Build history of the part. All positions in model axes, mm. A direction names the side the tool comes from. Round coordinates to 2 decimals unless told otherwise and drop trailing zeros. Loops run counter-clockwise (first coordinate to the right, second up) from the corner with the lowest first, then second, coordinate; pieces in that order, holes last.
Autodesk Inventor part; units mm, degrees
ref_plane "Arbeitsebene1" through (5, -3, 0) normal (0, 1, 0) x (-1, 0, 0)
ref_plane "YZ Plane" through (0, 0, 0) normal (1, 0, 0) x (0, 1, 0)
ref_plane "XY Plane" through (0, 0, 0) normal (0, 0, 1) x (1, 0, 0)
sketch "Skizze1" plane through (0, 0, 0) normal (0, 0, 1) x (1, 0, 0)
  line L0 (0, -0.6) -> (0, 3.6)
  line L1 (-2, 0) -> (12, 0)
  line L2 (0, 0) -> (10, 0)
  line L3 (10, 0) -> (10, 3)
  line L4 (10, 3) -> (0, 3)
  line L5 (0, 3) -> (0, 0)
  dimension "d1" = 10
  dimension "d2" = 6
revolve "Umdrehung1" add sketch "Skizze1" angle 360 about axis through (-10, 0, 0) along (1, 0, 0)
ref_plane "Arbeitsebene1" through (5, -3, 0) normal (0, 1, 0) x (-1, 0, 0)
sketch "Skizze2" plane through (5, -3, 0) normal (0, 1, 0) x (-1, 0, 0)
  line L0 (5, 3) -> (5, -3)
  line L1 (-5, 3) -> (-5, -3)
  line L2 (5, -3) -> (-5, -3)
  line L3 (5, 3) -> (-5, 3)
  line L4 (1.5, 3) -> (1.5, 1.5)
  line L5 (1.5, 1.5) -> (-5, 1.5)
  line L6 (-5, -1.5) -> (1.5, -1.5)
  line L7 (1.5, -1.5) -> (1.5, -3)
  line L8 (-5, 1.5) -> (-5, 3)
  line L9 (-5, 3) -> (1.5, 3)
  line L10 (-5, 3) -> (-5, -3)
  line L11 (-5, -1.5) -> (-5, -3)
  line L12 (-5, -3) -> (1.5, -3)
  dimension "d4" = 1.5
  dimension "d5" = 1.5
  dimension "d6" = 3.5
extrude "Extrusion1" cut sketch "Skizze2" along normal through all contours L4 L5 L1 L3 | L2 L1 L6 L7
chamfer "Fase1" distance 1.5 angle 33 1 edges at (0, -3, 0) measured on face at (4.5, -2.8079, -1.0563)
sketch "Skizze3" plane through (3.5, 2.5981, 1.5) normal (0, 0, 1) x (1, 0, 0)
  line L0 (6.5, 0) -> (6.5, -5.1962) construction
  arc A0 (3.5, -5.5981) -> (3.5, 0.4019) centre (3.5, -2.5981) ccw
  line L1 (6.5, 0) -> (6.5, 0.4019)
  line L2 (3.5, 0.4019) -> (7.092, 0.4019)
  line L3 (-2, 0.4019) -> (6.5, 0.4019)
  line L4 (7.092, 0.4019) -> (7.092, -5.5981)
  line L5 (7.092, -5.5981) -> (3.5, -5.5981)
  line L6 (-5.6184, -5.5981) -> (9.2105, -5.5981)
  point P0 (-3.5, -2.5981)
  point P1 (6.5, -5.5981)
  dimension "d13" = 3
  dimension "d14" = 3.592
extrude "Extrusion2" cut sketch "Skizze3" against normal through all
sketch "Skizze4" plane through (3.5, -2.5981, 1.5) normal (0, 0, 1) x (1, 0, 0)
  arc A0 (5, 0) -> (5, 5.1962) centre (3.5, 2.5981) ccw
  point P0 (-3.5, 2.5981)
hole "Bohrung1" at (7, 0, 1.5) at (7, 0, 1.5) direction (0, 0, -1) diameter 3 depth 3 tip angle 118
sketch "Skizze7" plane through (0, 0, 0) normal (-1, 0, 0) x (0, 0, 1)
  arc A0 (1.5, 2.5981) -> (-1.5, 2.5981) centre (0, 0) ccw
  circle A1 centre (0, 0) radius 3 construction
  line L0 (-1.5, 2.5981) -> (-1.5, 4)
  line L1 (-1.5, 4) -> (1.5, 4)
  line L2 (1.5, 4) -> (1.5, 2.5981)
  line L3 (0, -4.5424) -> (0, 5.5632)
  dimension "d25" = 1.5
  dimension "d26" = 3
  dimension "d27" = 4
sketch "Skizze8" plane through (3.5, -2.5981, 1.5) normal (0, 0, 1) x (1, 0, 0)
  line L0 (-2, 5.5981) -> (3.5, 5.5981)
  line L1 (3.5, 5.5981) -> (-3.5, 5.5981)
  arc A0 (5, 0) -> (5, 5.1962) centre (3.5, 2.5981) ccw
  arc A1 (3.5, -0.4019) -> (3.5, 5.5981) centre (3.5, 2.5981) ccw
  line L2 (-2, -0.4019) -> (3.5, -0.4019)
  line L3 (3.5, -0.4019) -> (-2.8962, -0.4019)
  point P0 (-3.5, 2.5981)
sweep "Sweeping2" cut profiles "Skizze7" path "Skizze8" path curves L1 A1 L3
sketch "Skizze9" plane through (0, 0, 0) normal (-1, 0, 0) x (0, 0, 1)
  point P0 (0, 0)
  point P1 (0, 0)
hole "Bohrung2" at (0, 0, 0) direction (1, 0, 0) diameter 2.459 depth 4 tip angle 118
properties part number "Stangenkopf"
(1) Slice it at C-C on x = 5. List the corners of the cut face in (y, z).
Responses:
outline: (-2.6, -1.5) - (2.6, -1.5) arc R3 ccw to (2.6, 1.5) - (-2.6, 1.5) arc R3 ccw to start
(2) Pull direction Y, two halves, no side cores. Call faces 4 (the face through (3.6, 2.86, -0.9)), 5 (the face through (2.028, 0.748, -0.976)), 6 (the face through (0, 1, -1)): +Y half, -Y half, draft (parallel to the pull), parting line (faces both ways), or undercut.
Responses:
face 4: parting line
face 5: undercut
face 6: draft
(3) Pin check, flat tips, straight feed: P1, Ø1.2, axis at y = 0.5, z = 2, coming from the +X side; P2, Ø2.5, axis at x = 6, y = -1, coming from the -Z side; P3, Ø3, axis at x = 8.5, z = -1, coming from the +Y side. Stop position of each tip, or through.
Responses:
P1: stops at x = 9.62
P2: stops at z = -1.5
P3: stops at y = 2.98
(4) Slice it at B-B on x = 2.5. List the corners of the cut face in (y, z).
Responses:
outline: circle Ø6 at (0, 0); hole circle Ø2.46 at (0, 0)
(5) Which spindle directions (+Z, -Z, +X, -X, +Y, -Y) get a long thin tool onto all of the face, cutting with end or side? Do faces 1 (the face through (4.61, 0.064, 0.204)), 2 (the face through (5, 0, 1.5)), 3 (the face through (5, 0, -1.5)). Say none if no direction does.
Responses:
face 1: -X
face 2: +Z, +X, +Y, -Y
face 3: -Z, +X, +Y, -Y
(6) Probe line 1 (Z direction, x = 2.65, y = 0); line 2 (Y direction, x = 7, z = -0.1). List the from-to ranges inside material, lowest first.
Responses:
line 1: z = -3 to -1.23, 1.23 to 3
line 2: y = -3 to -1.5, 1.5 to 3
